Could you check a few things on this model? Use its own coordinates, in mm. A direction names the side the tool comes from. Give positions to 0.01 mm unless a question says otherwise; leave off trailing zeros. Order: outer loops, then holes, each group sorted by start corner. A loop starts at its lowest first (then second) coordinate and runs counter-clockwise, first axis right, second up. Notation, with made-up numbers: M 33,-27.75 L 40,-27.75 A18 cw 40,4.25 Z; hole C 55.25,7 d4. An arc over 180 degrees is marked long. Use a Markdown table: item, result. Add a question column.
```python
from build123d import *

# Parameters (mm, degrees)
F3_R     = 6.35
F4_DEPTH = 5.08
F5_R     = 19.05
F5_R_2   = 6.35
F6_DEPTH = 2.54
F7_R     = 5.08
F8_DEPTH = 19.05


with BuildPart() as f2:
    # F1 (on Front) → F2 (revolve)
    with BuildSketch(Plane.XZ):
        Polygon((0, 25.4), (0, 0), (19.05, 0), align=None)
    revolve(axis=Axis((0, 0, 12.7), (0, 0, 1)))

    # F3 (on face) → F4 (join)
    with BuildSketch(Plane.XY):
        Circle(F3_R)
    extrude(amount=-F4_DEPTH)

    # F5 (on face) → F6 (join)
    with BuildSketch(Plane(origin=(0, 0, -5.08), x_dir=(1, 0, 0), z_dir=(0, 0, -1))):
        Circle(F5_R)
        Circle(F5_R_2, mode=Mode.SUBTRACT)
        Circle(F5_R_2)
    extrude(amount=F6_DEPTH)

    # F7 (on face) → F8 (cut)
    with BuildSketch(Plane(origin=(0, 0, -7.62), x_dir=(1, 0, 0), z_dir=(0, 0, -1))):
        Circle(F7_R)
    extrude(amount=-F8_DEPTH, mode=Mode.SUBTRACT)


solid = f2.part
```
1) Please list where these lines run through material, in increasing order: line 1 (Y direction, x = 0, z = -3); line 2 (Z direction, x = 0, y = 8.5); line 3 (Z direction, x = -1, y = 16). Write a range as from..to.
2) For pin 1 (1 mm diameter, centred on x = 7.5, y = 10.5, fed in from +Z); pin 2 (3 mm diameter, centred on y = 14.5, z = -4, fed in from -X); pin 3 (6 mm diameter, centred on x = 2.5, y = -3, fed in from +Z); pin 4 (1 mm diameter, centred on x = 10.5, z = 14.5, fed in from -Y), each with a flat end and sliding along its axis, tell me the tip position at first contact or that it passes through.
3) Suppose I cut it at A-A on z = 1. Please give me the cut outline in (x, y), and give its area (3 significant figures).
4) Suppose I cut it at B-B on z = 22. Please give me the cut outline in (x, y), and give its area (3 significant figures).
5) We'd pull the mould along Y, two halves only. Please class faces 1 (the face through (0, 0, 11.43)), 2 (the face through (5, 5, 0)), 3 (the face through (-15.12, 11.59, -6.33)): pulls with the +Y half, pulls with the -Y half, needs draft (parallel to the pull), parting line crosses it, or undercut.
6) For faces 4 (the face through (-5, -5, -5.08)), 5 (the face through (2.38, -4.58, 18.52)), 6 (the face through (-0.661, -5.037, 1.772)), which set-ups out of +Z, -Z, +X, -X, +Y, -Y let a thin tool reach every point of the face, with its end or its side?
7) Suppose I cut it at C-C on z = 18. Please give me the cut outline in (x, y).
Values found:
| question | item | result |
|---|---|---|
| 1 | line 1 | y = -6.35..-5.08, 5.08..6.35 |
| 1 | line 2 | z = -7.62..-5.08, 0..14.07 |
| 1 | line 3 | z = -7.62..-5.08, 0..4.03 |
| 2 | pin 1 | stops at z = 8.86 |
| 2 | pin 2 | stops at x = -13.48 |
| 2 | pin 3 | stops at z = 24.19 |
| 2 | pin 4 | passes through |
| 3 | outline | C 0,0 d36.6; hole C 0,0 d10.16 |
| 3 | area | 971 mm^2 |
| 4 | outline | C 0,0 d5.1 |
| 4 | area | 20.4 mm^2 |
| 5 | face 1 | undercut |
| 5 | face 2 | needs draft |
| 5 | face 3 | parting line crosses it |
| 6 | face 4 | none |
| 6 | face 5 | +Z |
| 6 | face 6 | -Z |
| 7 | outline | C 0,0 d11.1 |
